```python
from build123d import *

# Parameters (mm, degrees)
BOSS_EXTRUDE1_DEPTH = 35
SKETCH2_R           = 2.8
CUT_EXTRUDE1_DEPTH  = 10
CUT_EXTRUDE2_START  = -80
SKETCH2_2_R         = 2.8
CUT_EXTRUDE2_DEPTH  = 10


with BuildPart() as part:
    # Sketch1 → Boss-Extrude1 (new body)
    with BuildSketch(Plane(origin=(0, 0, 0), x_dir=(1, 0, 0), z_dir=(0, 1, 0))):
        with BuildLine():
            Line((-40, 17.5), (-40, -17.5))
            ThreePointArc((-40, -17.5), (0, -43.660622991), (40, -17.5))
            Line((40, -17.5), (40, 17.5))
            ThreePointArc((40, 17.5), (0, 43.660622991), (-40, 17.5))
        make_face()
    extrude(amount=BOSS_EXTRUDE1_DEPTH)

    # Sketch2 → Cut-Extrude1 (cut)
    with BuildSketch(Plane.ZY.offset(40)):
        with Locations((-11.5, 29)):
            Circle(SKETCH2_R)
        with Locations((11.5, 29)):
            Circle(SKETCH2_R)
        with Locations((-11.5, 6)):
            Circle(SKETCH2_R)
        with Locations((11.5, 6)):
            Circle(SKETCH2_R)
    extrude(amount=-CUT_EXTRUDE1_DEPTH, mode=Mode.SUBTRACT)

    # Sketch2<2> → Cut-Extrude2 (cut)
    with BuildSketch(Plane.ZY.offset(40).offset(CUT_EXTRUDE2_START)):
        with Locations((-11.5, 29)):
            Circle(SKETCH2_2_R)
        with Locations((11.5, 29)):
            Circle(SKETCH2_2_R)
        with Locations((-11.5, 6)):
            Circle(SKETCH2_2_R)
        with Locations((11.5, 6)):
            Circle(SKETCH2_2_R)
    extrude(amount=CUT_EXTRUDE2_DEPTH, mode=Mode.SUBTRACT)


solid = part.part
```
Build history of the part. All positions in model axes, mm. A direction names the side the tool comes from. Round coordinates to 2 decimals unless told otherwise and drop trailing zeros. Loops run counter-clockwise (first coordinate to the right, second up) from the corner with the lowest first, then second, coordinate; pieces in that order, holes last.
Item 1: Saw through at D-D (y = 21). List the corners of the cut face in (x, z).
Item 2: Saw through at A-A (z = -11.5). List the corners of the cut face in (x, y).
Item 3: Saw through at C-C (x = -24). List the corners of the cut face in (y, z).
Item 4: Pin check, flat tips, straight feed: P1, Ø4.5, axis at y = 29, z = -11.5, coming from the +X side; P2, Ø2, axis at x = -18, y = 20, coming from the +Z side; P3, Ø10, axis at y = 22.5, z = -31.5, coming from the -X side. Stop position of each tip, or through.
Item 5: Drill centre lines: line 1 along Y through (x, z) = (-36, -11.5); line 2 along X through (y, z) = (29.5, -9.5); line 3 along Z through (x, y) = (34.5, 31). Where is each one in solid material? Low to high.
Item 6: Saw through at B-B (y = 29). List the corners of the cut face in (x, z).
Item 7: Which spindle directions (+Z, -Z, +X, -X, +Y, -Y) get a long thin tool onto all of the face, cutting with end or side? Do faces 5 (the face through (-40, 17, 0)), 6 (the face through (30, 6, 11)), 7 (the face through (-30, 29, -12)). Say none if no direction does.
Item 8: Two-plate mould, pull along Z, no slides. Class faces 1 (the face through (-0.708, 17.255, 43.655)), 2 (the face through (0.708, 17.255, -43.655)), 3 (the face through (-1, 35, -1)), 4 (the face through (30, 6, -12)): released by +Z, released by -Z, zero draft, split by the parting line, or undercut.
Worked answers:
1. outline: (-40, -17.5) arc R43.66 ccw to (40, -17.5) - (40, 17.5) arc R43.66 ccw to (-40, 17.5) - close
2. outline: (-40, 0) - (40, 0) - (40, 3.2) - (30, 3.2) - (30, 8.8) - (40, 8.8) - (40, 26.2) - (30, 26.2) - (30, 31.8) - (40, 31.8) - (40, 35) - (-40, 35) - (-40, 31.8) - (-30, 31.8) - (-30, 26.2) - (-40, 26.2) - (-40, 8.8) - (-30, 8.8) - (-30, 3.2) - (-40, 3.2) - close
3. outline: (0, -36.47) - (35, -36.47) - (35, 36.47) - (0, 36.47) - close
4. P1: stops at x = 30
4. P2: stops at z = 40.22
4. P3: stops at x = -34.7
5. line 1: y = 0 to 3.2, 8.8 to 26.2, 31.8 to 35
5. line 2: x = -30 to 30
5. line 3: z = -26.76 to -13.46, -9.54 to 9.54, 13.46 to 26.76
6. outline: (-40, -17.5) arc R43.66 ccw to (40, -17.5) - (40, -14.3) - (30, -14.3) - (30, -8.7) - (40, -8.7) - (40, 8.7) - (30, 8.7) - (30, 14.3) - (40, 14.3) - (40, 17.5) arc R43.66 ccw to (-40, 17.5) - (-40, 14.3) - (-30, 14.3) - (-30, 8.7) - (-40, 8.7) - (-40, -8.7) - (-30, -8.7) - (-30, -14.3) - (-40, -14.3) - close
7. face 5: +Z, -Z, -X, +Y, -Y
7. face 6: +X
7. face 7: -X
8. face 1: released by +Z
8. face 2: released by -Z
8. face 3: zero draft
8. face 4: undercut
